Check sheet for the modelled part. Datum: model origin and axes. Units: mm. A direction names the side the tool comes from. Round coordinates to 2 decimals unless told otherwise and drop trailing zeros. Order: outer loops, then holes, each group sorted by start corner. A loop starts at its lowest first (then second) coordinate and runs counter-clockwise, first axis right, second up.
```python
from build123d import *

# Parameters (mm, degrees)
BOSS_EXTRUDE1_DEPTH          = 10
BOSS_EXTRUDE1_DEPTH_BACK     = 7
SKETCH1_W                    = 12
SKETCH1_H                    = 2
SKETCH1_W_2                  = 2.95
SKETCH1_H_2                  = 6.5
SKETCH1_3_W                  = 30
SKETCH1_3_H                  = 10
BOSS_EXTRUDE2_DEPTH          = 7
SKETCH3_W                    = 2.52297433
SKETCH3_H                    = 9
CUT_EXTRUDE1_DEPTH           = 34.823069051
M1_6X0_35_TAPPED_HOLE1_D     = 1.25
M1_6X0_35_TAPPED_HOLE1_DEPTH = 2.238512835
M1_6X0_35_TAPPED_HOLE2_D     = 1.25
M1_6X0_35_TAPPED_HOLE2_DEPTH = 2.95
F_1_5MM_DOWEL_HOLE1_D        = 1.5


with BuildPart() as part:
    # Sketch1 → Boss-Extrude1 (new, two sides: drawn at the far end of the back side and taken through both)
    with BuildSketch(Plane.XY.offset(-BOSS_EXTRUDE1_DEPTH_BACK)):
        with Locations((0, 1)):
            Rectangle(SKETCH1_W, SKETCH1_H)
        with Locations((4.525, -3.25)):
            Rectangle(SKETCH1_W_2, SKETCH1_H_2)
        with Locations((-4.525, -3.25)):
            Rectangle(SKETCH1_W_2, SKETCH1_H_2)
    extrude(amount=BOSS_EXTRUDE1_DEPTH + BOSS_EXTRUDE1_DEPTH_BACK)

    # Sketch1<3> → Boss-Extrude2 (add)
    with BuildSketch(Plane.XY):
        with Locations((0, 7)):
            Rectangle(SKETCH1_3_W, SKETCH1_3_H)
    extrude(amount=-BOSS_EXTRUDE2_DEPTH)

    # Sketch3 → Cut-Extrude1 (cut, through all)
    with BuildSketch(Plane.ZY.offset(15)):
        with Locations((-3.5, 7.5)):
            Rectangle(SKETCH3_W, SKETCH3_H)
    extrude(amount=-CUT_EXTRUDE1_DEPTH, mode=Mode.SUBTRACT)

    # M1.6x0.35 Tapped Hole1
    with Locations(Plane.XY):
        with Locations((6, 7), (-6, 7)):
            Hole(M1_6X0_35_TAPPED_HOLE1_D / 2, depth=M1_6X0_35_TAPPED_HOLE1_DEPTH)

    # M1.6x0.35 Tapped Hole2
    with Locations(Plane(origin=(6, 0, 0), x_dir=(0, 0, -1), z_dir=(1, 0, 0))):
        with Locations((3.5, -2.25), (-6.5, -2.25), (-1.5, -2.25)):
            Hole(M1_6X0_35_TAPPED_HOLE2_D / 2, depth=M1_6X0_35_TAPPED_HOLE2_DEPTH)

    # Ø1.5mm Dowel Hole1 (through all)
    with Locations(Plane.XY):
        with Locations((0, 7)):
            Hole(F_1_5MM_DOWEL_HOLE1_D / 2)


solid = part.part
```
Item 1: Scan lines: line 1 along Z through (x, y) = (-13.5, 7); line 2 along Y through (x, z) = (3.8, -3.5) (3 decimals); line 3 along X through (y, z) = (-4.5, -5.5). Record each from-to range of solid material in increasing order.
Answer:
line 1: z = -7 to -4.76, -2.24 to 0
line 2: y = -6.5 to -2.875, -1.625 to 3
line 3: x = -6 to -3.05, 3.05 to 6
Item 2: Sectioned sample at A-A (x = 0). Record the cut outline in (y, z).
Answer:
outline: (0, -7) - (6.25, -7) - (6.25, -4.76) - (3, -4.76) - (3, -2.24) - (6.25, -2.24) - (6.25, 0) - (2, 0) - (2, 10) - (0, 10) - close; (7.75, -7) - (12, -7) - (12, -4.76) - (7.75, -4.76) - close; (7.75, -2.24) - (12, -2.24) - (12, 0) - (7.75, 0) - close
Item 3: Release check for a two-part mould opening along X. For faces 1 (the flat face through (15, 7, -5)), 2 (the flat face through (-5, -6.5, 1)), 3 (the cylindrical face through (0.163, 6.268, -1.135)) record: released by +X, released by -X, zero draft, split by the parting line, or undercut.
Answer:
face 1: released by +X
face 2: zero draft
face 3: undercut
Item 4: Sectioned sample at D-D (y = -4). Record the cut outline in (x, z), and give its area (3 significant figures).
Answer:
outline: (-6, -7) - (-3.05, -7) - (-3.05, 10) - (-6, 10) - close; (3.05, -7) - (6, -7) - (6, 10) - (3.05, 10) - close
area: 100 mm2
Item 5: Sectioned sample at C-C (z = -3.5). Record the cut outline in (x, y) (3 decimals).
Answer:
outline: (-15, 2) - (-6, 2) - (-6, -6.5) - (-3.05, -6.5) - (-3.05, 0) - (3.05, 0) - (3.05, -1.625) - (6, -1.625) - (6, 2) - (15, 2) - (15, 3) - (-15, 3) - close; (3.05, -6.5) - (6, -6.5) - (6, -2.875) - (3.05, -2.875) - close
Item 6: Sectioned sample at B-B (y = 7). Record the cut outline in (x, z) (3 decimals).
Answer:
outline: (-15, -7) - (-0.75, -7) - (-0.75, -4.761) - (-15, -4.761) - close; (-15, -2.239) - (-6.625, -2.239) - (-6.625, 0) - (-15, 0) - close; (-5.375, -2.239) - (-0.75, -2.239) - (-0.75, 0) - (-5.375, 0) - close; (0.75, -7) - (15, -7) - (15, -4.761) - (0.75, -4.761) - close; (0.75, -2.239) - (5.375, -2.239) - (5.375, 0) - (0.75, 0) - close; (6.625, -2.239) - (15, -2.239) - (15, 0) - (6.625, 0) - close
Item 7: Access from +Z, -Z, +X, -X, +Y, -Y to the whole of each face (thin tool, end or side, straight path). Record for faces 4 (the flat face through (3.05, -3, 1)), 5 (the flat face through (0, 2, 5)), 6 (the cylindrical face through (-5.92, 7.62, -1.13)), 7 (the cylindrical face through (4.504, -2.63, -3.996)).
Answer:
face 4: +Z, -Z, -Y
face 5: +Z, +X, -X, +Y
face 6: +Z
face 7: +X
Item 8: Go/stop test with flat-tipped pins: P1, Ø1.1, axis at y = -2.25, z = 1.5, coming from the -X side; P2, Ø3, axis at y = 1.5, z = 1, coming from the -X side; P3, Ø2, axis at y = -2.25, z = 6.5, coming from the +X side; P4, Ø1.8, axis at x = -1.5, z = 3.5, coming from the -Y side. Record where each tip stops, or that it passes through.
Answer:
P1: stops at x = -6
P2: stops at x = -15
P3: stops at x = 6
P4: stops at y = 0
